Read the model definition and answer for the solid it produces. Units are mm, in the model's axes. A direction names the side the tool comes from. Coordinates: 2 decimals unless noted, no trailing zeros. Loops run counter-clockwise (first coordinate to the right, second up) from the corner with the lowest first, then second, coordinate; pieces in that order, holes last.
Q1. Section B-B (x = -4.75) is taken. Give the vertices of the cut face in (y, z), then the cut area to 3 significant figures.
Q2. Section C-C (z = 10) is taken. Give the vertices of the cut face in (x, y), then the cut area to 3 significant figures.
Q3. Section D-D (y = 27) is taken. Give the vertices of the cut face in (x, z).
Q4. Which of the six approach directions +Z, -Z, +X, -X, +Y, -Y give full straight-line access (tool end or side, diameter ignored) to faces 1 (the face through (0, 0, 30)), 2 (the face through (2.4, 27.1, 18.2))?
Q5. Flat-ended cylindrical pins translate along their axes: P1, Ø4, axis at x = -7.5, z = 19.5, coming from the +Y side; P2, Ø10, axis at x = -3, y = 46.5, coming from the -Z side; P3, Ø12, axis at y = 6.5, z = 4, coming from the -X side. Find the tip coordinate at first contact, or state that the pin passes through.
Q6. Section A-A (x = 0) is taken. Give the vertices of the cut face in (y, z).
Q7. Straight lines are drawn through the part: line 1 (Y direction, x = -3.5, z = 17); line 2 (Y direction, x = 8, z = 4.5); line 3 (Y direction, x = -4.5, z = 18.5). For each, find the intervals that lie inside material, in ascending order.
from build123d import *

# Parameters (mm, degrees)
SKETCH_1_R      = 10
EXTRUDE_2_DEPTH = 30
SKETCH_2_R      = 4
EXTRUDE_3_DEPTH = 50


with BuildPart() as part:
    # 草图1 → 凸台-拉伸2 (new body)
    with BuildSketch(Plane.XY):
        Circle(SKETCH_1_R)
    extrude(amount=EXTRUDE_2_DEPTH)

    # 草图2 → 凸台-拉伸3 (add)
    with BuildSketch(Plane(origin=(0, 0, 0), x_dir=(1, 0, 0), z_dir=(0, 1, 0))):
        with Locations(Location((0, -15, 0), (0, 0, 90))):
            Circle(SKETCH_2_R)
    extrude(amount=EXTRUDE_3_DEPTH)

    # 草图3 → 旋转1 (revolve)
    with BuildSketch(Plane(origin=(0, 50, 0), x_dir=(1, 0, 0), z_dir=(0, 1, 0))):
        with BuildLine():
            Line((0, -9), (0, -21))
            ThreePointArc((0, -21), (6, -15), (0, -9))
        make_face()
    revolve(axis=Axis((0, 50, 9), (0, 0, 1)))


solid = part.part
Numbers:
1. outline: (-8.8, 0) - (8.8, 0) - (8.8, 30) - (-8.8, 30) - close; circle Ø7.33 at (50, 15)
1. area: 570 mm2
2. outline: circle Ø20 at (0, 0); circle Ø6.63 at (0, 50)
2. area: 349 mm2
3. outline: circle Ø8 at (0, 15)
4. face 1: +Z, +X, -X, +Y, -Y
4. face 2: none
5. P1: stops at y = 8.35
5. P2: stops at z = 9
5. P3: stops at x = -9.99
6. outline: (-10, 0) - (10, 0) - (10, 11) - (45.53, 11) arc R6 ccw (long way) to (45.53, 19) - (10, 19) - (10, 30) - (-10, 30) - close
7. line 1: y = -9.37 to 9.37, 45.56 to 54.44
7. line 2: y = -6 to 6
7. line 3: y = -8.93 to 8.93, 48.13 to 51.87
